Study the drawing (mm; zero at the part's minimum x, y, z) and answer. A direction names the side the tool comes from. Round coordinates to 2 decimals unless told otherwise and drop trailing zeros. Loops run counter-clockwise (first coordinate to the right, second up) from the corner with the lowest first, then second, coordinate; pieces in that order, holes last. Notation, with made-up numbers: M 83.25,11 L 96.25,11 A33 ccw 96.25,49 Z; hole C 7,36.25 d1. An arc over 180 degrees is marked long. Put each result on its own line as item: value. Start each with the question number.
(1) Determine the mould class of the marked faces 5, 6 and 7 for opening direction X: released by +X, released by -X, zero draft, split by the parting line, or undercut.
(2) Flat-ended cylindrical pins translate along their axes: P1, Ø4, axis at y = 20.5, z = 23.5, coming from the +X side; P2, Ø8, axis at x = 16.5, y = 12.5, coming from the +Z side (1 decimal); P3, Ø10.5, axis at x = 4, z = 18.5, coming from the +Y side; P4, Ø12.5, axis at x = 25, y = 17, coming from the +Z side. Find the tip coordinate at first contact, or state that the pin passes through.
(3) Which of the six approach directions +Z, -Z, +X, -X, +Y, -Y give full straight-line access (tool end or side, diameter ignored) to the marked faces 1, 2, 3 and 4?
(4) Section C-C, the plane z = 29 is taken. Count the separate pieces of the cut face and the enclosed holes in it.
(5) Section B-B, the plane x = 19 is taken. Determine the outline of the cut face in (y, z) (1 decimal).
(6) Section A-A, the plane y = 17 is taken. Determine the outline of the cut face in (x, z) (1 decimal), then the cut area to 3 significant figures.
(7) Straight lines are drawn through the part: line 1 (Y direction, x = 44, z = 14.5); line 2 (X direction, y = 16, z = 32) (1 decimal); line 3 (Y direction, x = 18, z = 20) (1 decimal). For each, find the intervals that lie inside material, in ascending order.
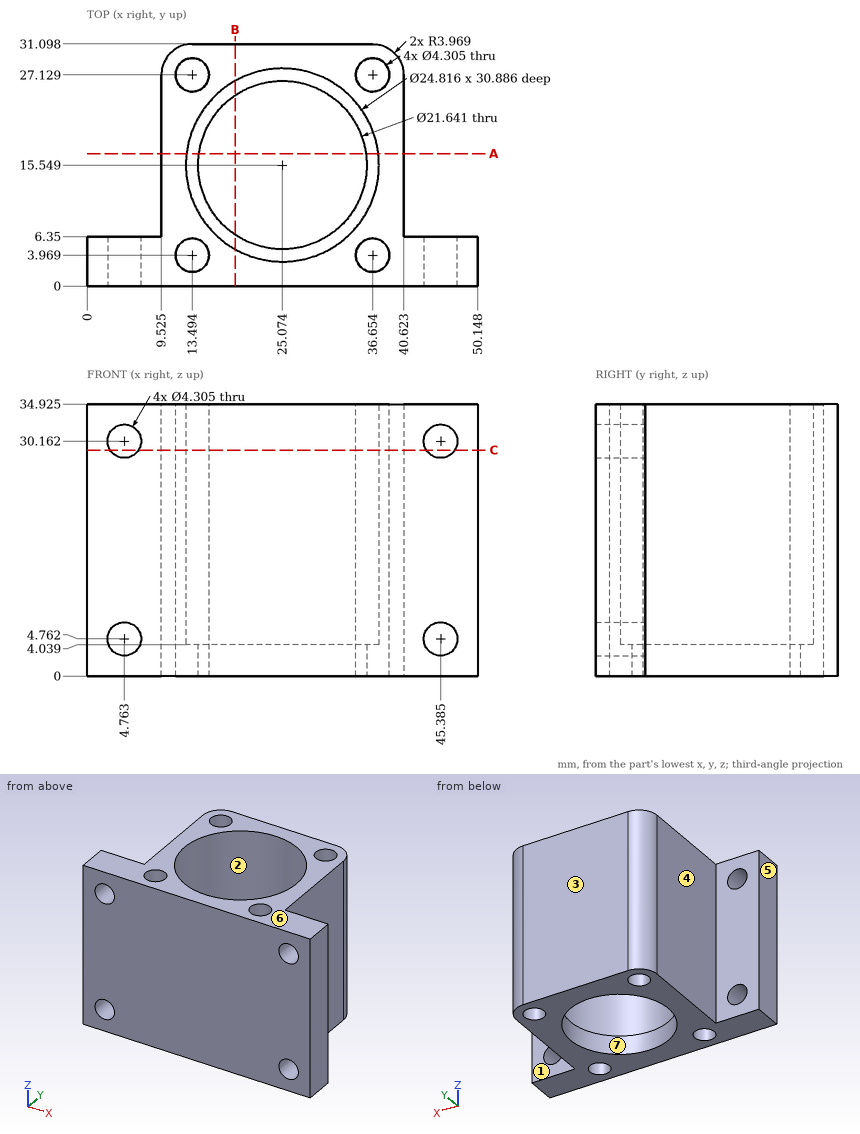
Recorded:
1. face 5: released by -X
1. face 6: zero draft
1. face 7: undercut
2. P1: stops at x = 40.62
2. P2: stops at z = 34.9
2. P3: stops at y = 6.35
2. P4: passes through
3. face 1: +Z, -Z, +X, +Y
3. face 2: +Z
3. face 3: +Z, -Z, +X, -X, +Y
3. face 4: +Z, -Z, -X, +Y
4. separate pieces: 3
4. enclosed holes: 5
5. outline: M 0,0 L 6.6,0 L 6.6,4 L 4.7,4 L 4.7,34.9 L 0,34.9 Z; M 24.5,0 L 31.1,0 L 31.1,34.9 L 26.4,34.9 L 26.4,4 L 24.5,4 Z
6. outline: M 9.5,0 L 14.4,0 L 14.4,4 L 12.8,4 L 12.8,34.9 L 9.5,34.9 Z; M 35.8,0 L 40.6,0 L 40.6,34.9 L 37.4,34.9 L 37.4,4 L 35.8,4 Z
6. area: 238 mm²
7. line 1: y = 0 to 6.35
7. line 2: x = 9.5 to 12.7, 37.5 to 40.6
7. line 3: y = 0 to 5.4, 25.7 to 31.1
